Drawing for the job (mm, zero at the part's lowest x, y, z). A direction names the side the tool comes from. Coordinates: 2 decimals unless noted, no trailing zeros. Write each loop counter-clockwise with the first axis right and the second up, starting at its lowest first coordinate (ties: lowest second). Pieces come first, ordered by that corner, then holes. Notation, with made-up numbers: M -33.5,8.25 L 17.5,8.25 A25 ccw 17.5,40.25 Z; hole C -16.75,84 d2. An arc over 180 degrees is marked long. Put each result on its own line as item: value. Start each with the question number.
Q1. Drill centre lines: line 1 along Y through (x, z) = (14.5, 11); line 2 along X through (y, z) = (3.05, 7) (1 decimal); line 3 along Z through (x, y) = (7.75, 1.65). Where is each one in solid material? Low to high.
Q2. Drop flat-ended pins along their axis: pin 1 (5 mm diameter, centred on x = 10.5, z = 3, fed in from +Y); pin 2 (2 mm diameter, centred on x = 7, z = 7.5, fed in from +Y); pin 3 (2 mm diameter, centred on y = 3.5, z = 10, fed in from -X); pin 4 (1 mm diameter, centred on x = 8, y = 3.5, fed in from +Z). Give the stop position or say it passes through.
Q3. Cut at B-B (y = 1.05). Write the cut outline in (x, z).
Q4. Cut at D-D (z = 14.75). Write the cut outline in (x, y).
Q5. Cut at A-A (x = 8). Write the cut outline in (y, z), then the cut area to 3 significant figures.
Q6. Cut at C-C (z = 11.75). Write the cut outline in (x, y).
Q7. Which spindle directions (+Z, -Z, +X, -X, +Y, -Y) get a long thin tool onto all of the face, cutting with end or side? Do the marked faces 1 and 2. Say none if no direction does.
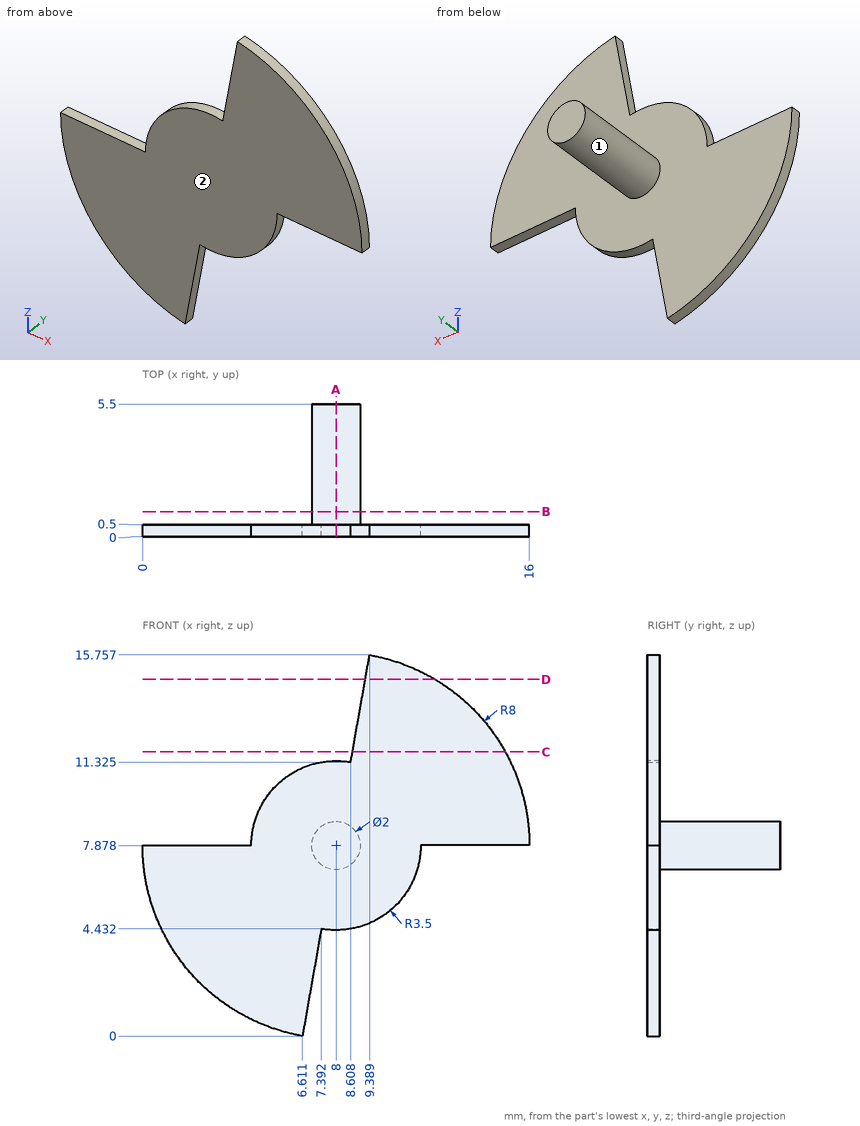
Computed values:
1. line 1: 0 to 0.5
1. line 2: 7.5 to 8.5
1. line 3: 6.91 to 8.85
2. pin 1: y = 0.5
2. pin 2: y = 5.5
2. pin 3: through
2. pin 4: z = 8.88
3. outline: C 8,7.88 d2
4. outline: M 9.21,0 L 12.1,0 L 12.1,0.5 L 9.21,0.5 Z
5. outline: M 0,4.38 L 0.5,4.38 L 0.5,6.88 L 5.5,6.88 L 5.5,8.88 L 0.5,8.88 L 0.5,11.38 L 0,11.38 Z
5. area: 13.5 mm2
6. outline: M 8.68,0 L 15,0 L 15,0.5 L 8.68,0.5 Z
7. face 1: +Y
7. face 2: +Z, -Z, +X, -X, -Y
